Geometry check sheet. Reference: the model listing, model coordinates, mm. A direction names the side the tool comes from. Coordinates: 2 decimals unless noted, no trailing zeros. Order: outer loops, then holes, each group sorted by start corner. A loop starts at its lowest first (then second) coordinate and runs counter-clockwise, first axis right, second up. Notation, with made-up numbers: M -21.5,-39.75 L 33.5,-39.75 A5 cw 33.5,-33.75 Z; hole C -13.75,70 d9. An arc over 180 degrees is marked long. One line per item, written item: value. Start each with the question number.
1) Access from +Z, -Z, +X, -X, +Y, -Y to the whole of each face (thin tool, end or side, straight path). Record for faces 5 (the flat face through (-59, 0, 63)), 6 (the flat face through (-328.64, -125.22, -134.75)), 7 (the flat face through (-287.1, -125.2, -184.1)), 8 (the flat face through (-59, -254, 63)), 9 (the flat face through (59.265, -125.222, -195.778)).
2) Thickness scan on L1, parallel to X at y = -52, z = -97.5; L2, parallel to Z at x = -394, y = -85; L3, parallel to X at y = -34.5, z = -252. Record the ranges inside material, lowest first. Write a range as from..to.
3) Draft check along Z on faces 1 (the flat face through (185.271, -125.222, 19.963)), 2 (the flat face through (-327.43, -125.22, 57.19)), 3 (the flat face through (-93.164, -125.222, 270.292)), 4 (the flat face through (-10, -125, -204)). Enter one of: pulls with the +Z half, pulls with the -Z half, needs draft (parallel to the pull), parting line crosses it, or undercut.
4) Sectioned sample at D-D, the plane x = 268. Enter the section's corners in (y, z).
5) Go/stop test with flat-tipped pins: P1, Ø3, axis at x = -335, y = -178.5, coming from the +Z side; P2, Ø4, axis at x = 25, y = -106, coming from the -Z side; P3, Ø6, axis at x = 35, z = -9.5, coming from the +Y side; P4, Ø4, axis at x = 185.5, y = -70.5, coming from the +Z side. Record where each tip stops, or that it passes through.
6) Sectioned sample at B-B, the plane x = -367. Enter the section's corners in (y, z).
7) Sectioned sample at C-C, the plane z = 123. Enter the section's corners in (x, y).
8) Sectioned sample at A-A, the plane y = -98.5. Enter the section's corners in (x, z).
```python
from build123d import *

# Parameters (mm, degrees)
F1_DEPTH = 254


with BuildPart() as f1:
    # F0 (on Front) → F1 (new body)
    with BuildSketch(Plane.XZ):
        with BuildLine():
            ThreePointArc((-162.177067, 149.106595), (-54.889921, 188.841494), (47.638746, 138.074711))
            Line((47.638746, 138.074711), (-26.05729, 388.13132))
            Line((-26.05729, 388.13132), (-162.177067, 149.106595))
        make_face()
        with BuildLine():
            Line((-461.089432, -273.319095), (-108.239205, -92.380688))
            ThreePointArc((-108.239205, -92.380688), (-165.032116, -57.088534), (-199.844044, 0))
            Line((-199.844044, 0), (-461.089432, -273.319095))
        make_face()
        with BuildLine():
            ThreePointArc((47.638746, 138.074711), (73.107329, 94.392598), (81.95847, 44.608735))
            ThreePointArc((81.95847, 44.608735), (21.937886, -72.589023), (-108.239205, -92.380688))
            Line((-108.239205, -92.380688), (90.14336, -317.783058))
            Line((90.14336, -317.783058), (27.508762, -70.308436))
            Line((27.508762, -70.308436), (347.513378, 112.797849))
            Line((347.513378, 112.797849), (47.638746, 138.074711))
        make_face()
        with BuildLine():
            ThreePointArc((-108.239205, -92.380688), (21.937886, -72.589023), (81.95847, 44.608735))
            ThreePointArc((81.95847, 44.608735), (73.107329, 94.392598), (47.638746, 138.074711))
            ThreePointArc((47.638746, 138.074711), (-54.889921, 188.841494), (-162.177067, 149.106595))
            ThreePointArc((-162.177067, 149.106595), (-202.506455, 79.983544), (-199.844044, 0))
            ThreePointArc((-199.844044, 0), (-165.032116, -57.088534), (-108.239205, -92.380688))
        make_face()
        with BuildLine():
            ThreePointArc((-199.844044, 0), (-202.506455, 79.983544), (-162.177067, 149.106595))
            Line((-162.177067, 149.106595), (-451.486111, 112.797849))
            Line((-451.486111, 112.797849), (-199.844044, 0))
        make_face()
    extrude(amount=F1_DEPTH)


solid = f1.part
```
Final values:
1. face 5: +Z, -Z, +X, -X, +Y
1. face 6: -X, +Y, -Y
1. face 7: -Z, +Y, -Y
1. face 8: +Z, -Z, +X, -X, -Y
1. face 9: +X, +Y, -Y
2. L1: x = -293.04..-118.22, -103.73..34.39
2. L2: z = -238.92..-203.13, 87.03..120.01
2. L3: x = -440.71..-419.51, 32.25..73.49
3. face 1: undercut
3. face 2: undercut
3. face 3: pulls with the +Z half
3. face 4: pulls with the -Z half
4. outline: M -254,67.3 L 0,67.3 L 0,119.5 L -254,119.5 Z
5. P1: stops at z = 127.61
5. P2: stops at z = -246.04
5. P3: stops at y = 0
5. P4: stops at z = 126.62
6. outline: M -254,-225.07 L 0,-225.07 L 0,-174.88 L -254,-174.88 Z; M -254,74.93 L 0,74.93 L 0,123.4 L -254,123.4 Z
7. outline: M -370.2,-254 L 226.48,-254 L 226.48,0 L -370.2,0 Z
8. outline: M -461.09,-273.32 L -108.24,-92.38 L 90.14,-317.78 L 27.51,-70.31 L 347.51,112.8 L 47.64,138.07 L -26.06,388.13 L -162.18,149.11 L -451.49,112.8 L -199.84,0 Z
